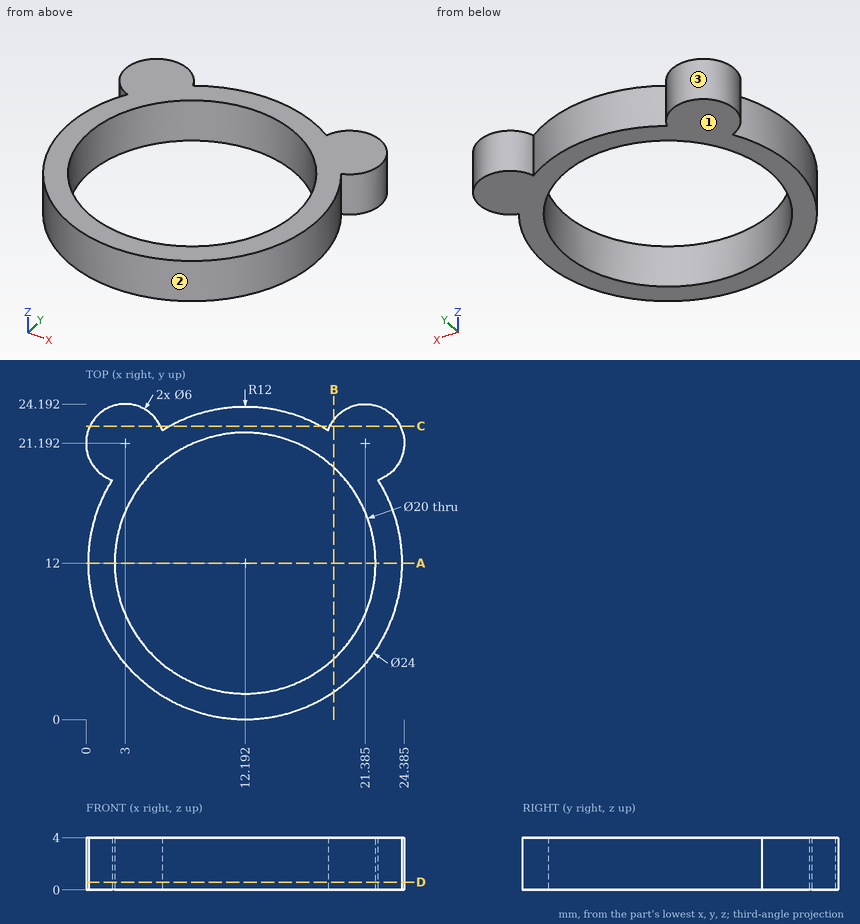
Print and shaded views of the part. All mm, measured from the part's lowest x, y and z. Give positions to 0.01 mm unless a question says otherwise; leave off trailing zeros. Order: outer loops, then holes, each group sorted by start corner. A loop starts at its lowest first (then second) coordinate and runs counter-clockwise, first axis right, second up. Notation, with made-up numbers: M 74.5,89 L 84.5,89 A25 ccw 84.5,106 Z; hole C 84,37 d6. An arc over 180 degrees is marked long. Use one line per item in the form item = value.
Q1. Slice it at D-D, the plane z = 0.6. Write the cut outline in (x, y) (1 decimal).
Conclusion:
outline = M 2,18.4 A12 ccw long 22.4,18.4 A3 ccw long 18.6,22.2 A12 ccw 5.8,22.2 A3 ccw long Z; hole C 12.2,12 d20
Q2. Wall check: probe 1 along Y at (x, z) = (12.25, 0.7); probe 2 along X at (y, z) = (12.25, 0.35) (1 decimal); probe 3 along Y at (x, z) = (22.75, 3.3) (1 decimal). Give the ranges that are in metal, low to high.
Conclusion:
probe_1 = 0 to 2, 22 to 24
probe_2 = 0.2 to 2.2, 22.2 to 24.2
probe_3 = 6.3 to 17.7, 18.5 to 23.9
Q3. Pin check, flat tip, straight feed: P1, Ø2, axis at x = 4, y = 6.5, coming from the -Z side. Stop position of the tip, or through.
Conclusion:
P1 = 0
Q4. Slice it at C-C, the plane y = 22.5. Write the cut outline in (x, z) (1 decimal).
Conclusion:
outline = M 0.3,0 L 5.7,0 L 5.7,4 L 0.3,4 Z; M 6.4,0 L 18,0 L 18,4 L 6.4,4 Z; M 18.7,0 L 24.1,0 L 24.1,4 L 18.7,4 Z
Q5. Slice it at B-B, the plane x = 19. Write the cut outline in (y, z) (1 decimal).
Conclusion:
outline = M 2.1,0 L 4.7,0 L 4.7,4 L 2.1,4 Z; M 19.3,0 L 23,0 L 23,4 L 19.3,4 Z
Q6. Slice it at A-A, the plane y = 12. Write the cut outline in (x, z), and give its area (3 significant figures).
Conclusion:
outline = M 0.19,0 L 2.19,0 L 2.19,4 L 0.19,4 Z; M 22.19,0 L 24.19,0 L 24.19,4 L 22.19,4 Z
area = 16.0 mm2
Q7. Pull direction X, two halves, no side cores. Call the marked faces 1, 2 and 3: released by +X, released by -X, zero draft, split by the parting line, or undercut.
Conclusion:
face_1 = zero draft
face_2 = split by the parting line
face_3 = undercut
